```python
from build123d import *

# Parameters (mm, degrees)
SKETCH_3_R          = 8
EXTRUDE_1_DEPTH     = 5
SKETCH_4_R          = 4
CUT_EXTRUDE_1_DEPTH = 213.248558243


with BuildPart() as part:
    # 草图3 → 凸台-拉伸1 (new body)
    with BuildSketch(Plane.XY):
        with BuildLine():
            ThreePointArc((203.259167971, -8.750002099), (194.509167971, -2.099e-06), (203.259167971, 8.749997901))
            Line((203.259167971, 8.749997901), (0, 8.749997901))
            Line((0, 8.749997901), (-11.740832029, 8))
            ThreePointArc((-11.740832029, 8), (-6.08397778, 5.656854249), (-3.740832029, 0))
            ThreePointArc((-3.740832029, 0), (-6.08397778, -5.656854249), (-11.740832029, -8))
            Line((-11.740832029, -8), (0, -8.750038444))
            Line((0, -8.750038444), (203.259167971, -8.750002099))
        make_face()
        with Locations((-11.740832029, 0)):
            Circle(SKETCH_3_R)
        with BuildLine():
            ThreePointArc((212.009167971, -2.099e-06), (209.446352306, 6.187182236), (203.259167971, 8.749997901))
            Line((203.259167971, 8.749997901), (203.259167971, -8.750002099))
            ThreePointArc((203.259167971, -8.750002099), (209.446352306, -6.187186435), (212.009167971, -2.099e-06))
        make_face()
        with BuildLine():
            Line((203.259167971, -8.750002099), (203.259167971, 8.749997901))
            ThreePointArc((203.259167971, 8.749997901), (194.509167971, -2.099e-06), (203.259167971, -8.750002099))
        make_face()
    extrude(amount=EXTRUDE_1_DEPTH)

    # 草图4 → 切除-拉伸1 (cut, through all)
    with BuildSketch(Plane.XY.offset(5)):
        with Locations((-11.740832029, 0)):
            Circle(SKETCH_4_R)
        with Locations((203.259167971, -2.099e-06)):
            Circle(SKETCH_4_R)
    extrude(amount=-CUT_EXTRUDE_1_DEPTH, mode=Mode.SUBTRACT)


solid = part.part
```
Geometry check sheet. Reference: the model listing, model coordinates, mm. Coordinates: 2 decimals unless noted, no trailing zeros. Loops run counter-clockwise (first coordinate to the right, second up) from the corner with the lowest first, then second, coordinate; pieces in that order, holes last.
Item 1: Thickness scan on line 1 (X direction, y = 3, z = 0.35); line 2 (X direction, y = 1.25, z = 2.6); line 3 (X direction, y = 6, z = 2.1). Record the ranges inside material, lowest first.
Item 2: Sectioned sample at A-A, the plane z = 1.55. Record the boundary of the cut face in (x, y).
Item 3: Go/stop test with flat-tipped pins: pin 1 Ø3 at (y, z) = (-5.5, 1.5) entering from -X; pin 2 Ø2 at (y, z) = (5.5, 2) entering from -X; pin 3 Ø9 at (x, y) = (-11.74, 0) entering from -Z. Record where each tip stops, or that it passes through.
Item 4: Release check for a two-part mould opening along Y. For faces 1 (the face through (103, 8.75, 2)), 2 (the face through (207.074, 1.201, 2.535)), 3 (the face through (95, 0, 0)), 4 (the face through (-9.9, -3.55, 2.54)) record: released by +Y, released by -Y, zero draft, split by the parting line, or undercut.
Check result:
1. line 1: x = -19.16 to -14.39, -9.1 to 200.61, 205.9 to 211.48
1. line 2: x = -19.64 to -15.54, -7.94 to 199.46, 207.06 to 211.92
1. line 3: x = -17.03 to 209.63
2. outline: (-11.74, -8) - (0, -8.75) - (203.26, -8.75) arc R8.75 ccw to (203.26, 8.75) - (0, 8.75) - (-11.74, 8) arc R8 ccw to start; hole circle Ø8 at (-11.74, 0); hole circle Ø8 at (203.26, 0)
3. pin 1: stops at x = -18.67
3. pin 2: stops at x = -18.36
3. pin 3: stops at z = 0
4. face 1: released by +Y
4. face 2: undercut
4. face 3: zero draft
4. face 4: undercut
